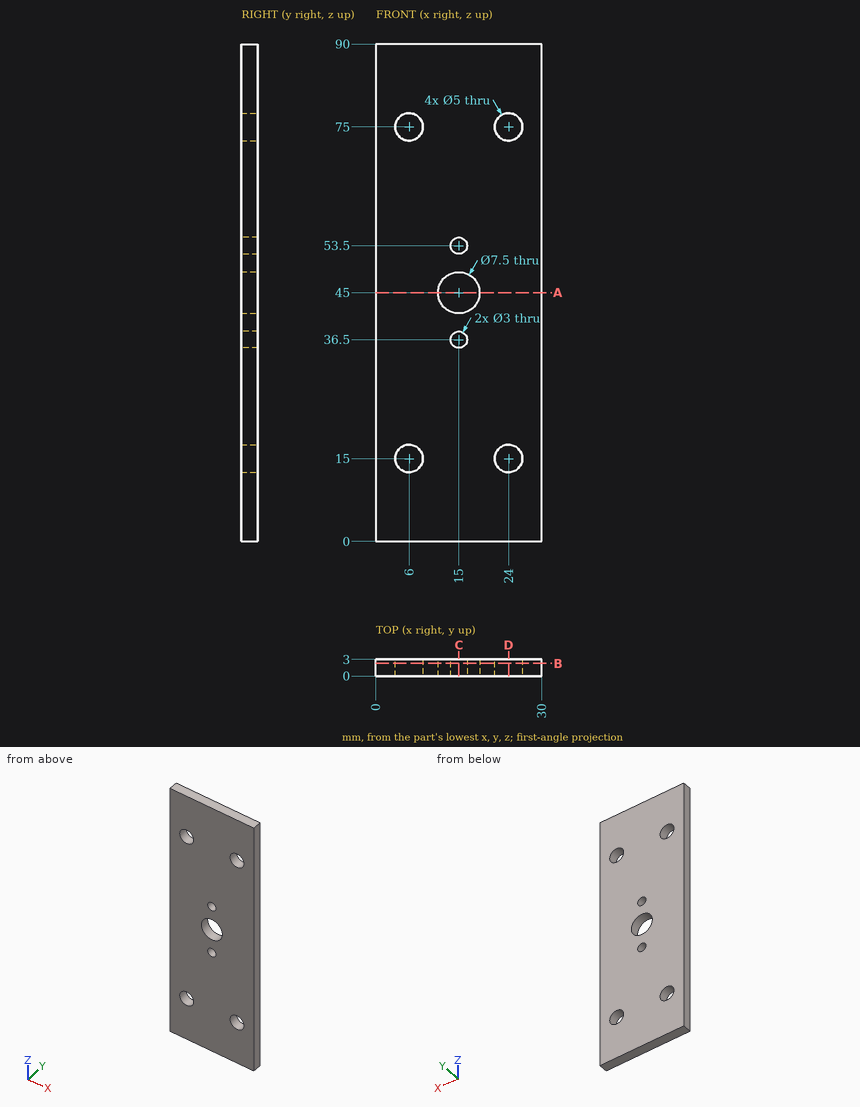
Check sheet for the drawn part. Datum: minimum x, y, z corner. Units: mm. Round coordinates to 2 decimals unless told otherwise and drop trailing zeros. Order: outer loops, then holes, each group sorted by start corner. A loop starts at its lowest first (then second) coordinate and runs counter-clockwise, first axis right, second up.
1. Go/stop test with a flat-tipped pin: P1, Ø3, axis at x = 6, z = 75, coming from the +Y side. Record where the tip stops, or that it passes through.
Final values:
P1: passes through
2. Section check D-D on x = 24. Record the cut outline in (y, z), then the cut area to 3 significant figures.
Final values:
outline: (0, 0) - (3, 0) - (3, 12.5) - (0, 12.5) - close; (0, 17.5) - (3, 17.5) - (3, 72.5) - (0, 72.5) - close; (0, 77.5) - (3, 77.5) - (3, 90) - (0, 90) - close
area: 240 mm2
3. Section check C-C on x = 15. Record the cut outline in (y, z).
Final values:
outline: (0, 0) - (3, 0) - (3, 35) - (0, 35) - close; (0, 38) - (3, 38) - (3, 41.25) - (0, 41.25) - close; (0, 48.75) - (3, 48.75) - (3, 52) - (0, 52) - close; (0, 55) - (3, 55) - (3, 90) - (0, 90) - close
4. Section check A-A on z = 45. Record the cut outline in (x, y), then the cut area to 3 significant figures.
Final values:
outline: (0, 0) - (11.25, 0) - (11.25, 3) - (0, 3) - close; (18.75, 0) - (30, 0) - (30, 3) - (18.75, 3) - close
area: 67.5 mm2
5. Section check B-B on y = 2.3. Record the cut outline in (x, z).
Final values:
outline: (0, 0) - (30, 0) - (30, 90) - (0, 90) - close; hole circle Ø5 at (6, 15); hole circle Ø5 at (6, 75); hole circle Ø7.5 at (15, 45); hole circle Ø3 at (15, 36.5); hole circle Ø3 at (15, 53.5); hole circle Ø5 at (24, 15); hole circle Ø5 at (24, 75)
6. Thickness scan on L1, parallel to X at y = 1.2, z = 75; L2, parallel to Z at x = 24, y = 0.85; L3, parallel to Z at x = 15, y = 1.2. Record the ranges inside material, lowest first.
Final values:
L1: x = 0 to 3.5, 8.5 to 21.5, 26.5 to 30
L2: z = 0 to 12.5, 17.5 to 72.5, 77.5 to 90
L3: z = 0 to 35, 38 to 41.25, 48.75 to 52, 55 to 90
